Source: CAD feature listing. Evaluate the final solid. Frame: model axes, mm. A direction names the side the tool comes from. Give positions to 0.01 mm unless a question says otherwise; leave off trailing zeros. Answer as CSV lines item,"result".
```python
from build123d import *

# Parameters (mm, degrees)
BOSS_EXTRUDE1_DEPTH      = 304.8
F_1_4_CLEARANCE_HOLE1_D  = 6.7564
F_1_4_CLEARANCE_HOLE2_D  = 6.7564
F_5_16_CLEARANCE_HOLE1_D = 8.4328


with BuildPart() as part:
    # Sketch2 → Boss-Extrude1 (new, symmetric)
    with BuildSketch(Plane.XY):
        with BuildLine():
            Line((-12.7, -12.7), (12.7, -12.7))
            Line((12.7, -12.7), (12.7, 12.7))
            Line((12.7, 12.7), (11.1125, 12.7))
            ThreePointArc((11.1125, 12.7), (9.989967985, 12.235032015), (9.525, 11.1125))
            Line((9.525, 11.1125), (9.525, -6.35))
            ThreePointArc((9.525, -6.35), (8.59506403, -8.59506403), (6.35, -9.525))
            Line((6.35, -9.525), (-11.1125, -9.525))
            ThreePointArc((-11.1125, -9.525), (-12.235032015, -9.989967985), (-12.7, -11.1125))
            Line((-12.7, -11.1125), (-12.7, -12.7))
        make_face()
    extrude(amount=BOSS_EXTRUDE1_DEPTH, both=True)

    # 1/4 Clearance Hole1 (through all)
    with Locations(Plane(origin=(0, -9.525, 0), x_dir=(-1, 0, 0), z_dir=(0, 1, 0))):
        with Locations((2.38125, 282.575), (2.38125, -228.6), (2.38125, 105.9688)):
            Hole(F_1_4_CLEARANCE_HOLE1_D / 2)

    # 1/4 Clearance Hole2 (through all)
    with Locations(Plane.ZY.offset(-9.525)):
        with Locations((254, 2.38125), (190.5, 2.38125), (127, 2.38125), (63.5, 2.38125)):
            Hole(F_1_4_CLEARANCE_HOLE2_D / 2)

    # 5/16 Clearance Hole1 (through all)
    with Locations(Plane(origin=(0, -9.525, 0), x_dir=(1, 0, 0), z_dir=(0, 1, 0))):
        with Locations((-2.38125, 279.4)):
            Hole(F_5_16_CLEARANCE_HOLE1_D / 2)


solid = part.part
```
(1) Access query for faces 1 (the flat face through (6, -10, 304.8)), 2 (the flat face through (-2, -9.525, 4)). Directions: +Z, -Z, +X, -X, +Y, -Y. A direction counts if a zero-diameter tool reaches every point of the face in a straight line with its end or side. Return the directions, or none.
Completed:
face 1,"+Z, +X, -X, +Y, -Y"
face 2,"+Z, -Z, -X, +Y"
(2) Contact query for flat-ended pins moving along their axis: pin 1 (8.5 mm diameter, centred on x = -5.5, z = 108.5, fed in from +Y) (3 decimals); pin 2 (5 mm diameter, centred on y = 5, z = -174, fed in from -X) (3 decimals); pin 3 (5.5 mm diameter, centred on x = -2.38, z = 105.97, fed in from +Y); pin 4 (8 mm diameter, centred on y = -6.5, z = 136.5, fed in from -X). Output: stop coordinate, or through.
Completed:
pin 1,"y = -9.525"
pin 2,"x = 9.525"
pin 3,"through"
pin 4,"x = -12.58"
(3) Ray query, line 1 (Y direction, x = 12.05, z = 127); line 2 (X direction, y = -11.2, z = -228.6); line 3 (X direction, y = 10, z = -178) (3 decimals). Return the intervals inside material, ascending. Write a range as from..to.
Completed:
line 1,"-12.7..-1, 5.76..12.7"
line 2,"-12.7..-5.76, 1..12.7"
line 3,"9.525..12.7"
